from build123d import *

# Parameters (mm, degrees)
SKETCH018_W     = 50
SKETCH018_H     = 18
PAD011_DEPTH    = 4.5
SKETCH019_R     = 1.3375
POCKET006_DEPTH = 8
POCKET007_DEPTH = 9.001
SKETCH053_R     = 1.3375
SKETCH053_R_2   = 2.5
PAD029_DEPTH    = 6.5
SKETCH055_W     = 8.5
SKETCH055_H     = 1
SKETCH055_W_2   = 24
POCKET024_DEPTH = 1


with BuildPart() as part:
    # Sketch018 → Pad011 (new body, symmetric)
    with BuildSketch(Plane.XY):
        with Locations((25, 9)):
            Rectangle(SKETCH018_W, SKETCH018_H)
    extrude(amount=PAD011_DEPTH, both=True)

    # Sketch019 → Pocket006 (cut)
    with BuildSketch(Plane.XZ):
        with Locations((5, 0)):
            Circle(SKETCH019_R)
        with Locations((25, 0)):
            Circle(SKETCH019_R)
        with Locations((45, 0)):
            Circle(SKETCH019_R)
    extrude(amount=-POCKET006_DEPTH, mode=Mode.SUBTRACT)

    # Sketch020 (on Face4 of Pocket006) → Pocket007 (cut, through all)
    with BuildSketch(Plane(origin=(0, 0, -4.5), x_dir=(1, 0, 0), z_dir=(0, 0, -1))):
        Polygon((0, -8), (43.5, -18), (0, -18), align=None)
    extrude(amount=-POCKET007_DEPTH, mode=Mode.SUBTRACT)

    # Sketch053 → Pad029 (join)
    with BuildSketch(Plane.YZ.offset(50)):
        Polygon((18, -4.5), (-6.5, -4.5), (-6.5, 4.5), (-15.5, 4.5), (-15.5, -4.5), (0, -24.5), (18, -24.5), align=None)
        with Locations((14, -7)):
            Circle(SKETCH053_R, mode=Mode.SUBTRACT)
        with Locations((4, -7)):
            Circle(SKETCH053_R, mode=Mode.SUBTRACT)
        with Locations((4, -22)):
            Circle(SKETCH053_R, mode=Mode.SUBTRACT)
        with Locations((14, -22)):
            Circle(SKETCH053_R, mode=Mode.SUBTRACT)
        with Locations((-11, 0)):
            Circle(SKETCH053_R_2, mode=Mode.SUBTRACT)
    extrude(amount=-PAD029_DEPTH)

    # Sketch055 (on Face7 of Pad029) → Pocket024 (cut)
    with BuildSketch(Plane.YZ.offset(50)):
        with Locations((13.75, -14.5)):
            Rectangle(SKETCH055_W, SKETCH055_H)
        with Locations((-3.5, -14.5)):
            Rectangle(SKETCH055_W_2, SKETCH055_H)
    extrude(amount=-POCKET024_DEPTH, mode=Mode.SUBTRACT)


with BuildPart() as part_1:
    # Body005 placement: moved
    add(part.part.moved(Location((75, 6.5, 0))))


solid = part_1.part
Work out the finished part from the listing and answer in its coordinate system (mm). A direction names the side the tool comes from. Coordinates: 2 decimals unless noted, no trailing zeros. Write each loop counter-clockwise with the first axis right and the second up, starting at its lowest first coordinate (ties: lowest second). Pieces come first, ordered by that corner, then holes. Notation, with made-up numbers: M 20.25,7.5 L 25.25,7.5 A33 ccw 25.25,40.5 Z; hole C -25,59 d1. An arc over 180 degrees is marked long. Write item = value, one per line.
1. The part is cut by section D-D (x = 120). Determine the outline of the cut face in (y, z) (1 decimal), then the cut area to 3 significant figures.
Solution:
outline = M -9,-4.5 L 6.5,-24.5 L 24.5,-24.5 L 24.5,4.5 L 6.5,4.5 L 6.5,1.3 L 14.5,1.3 L 14.5,-1.3 L 6.5,-1.3 L 6.5,-4.5 L 0,-4.5 L 0,4.5 L -9,4.5 Z; hole C -4.5,0 d5; hole C 10.5,-22 d2.7; hole C 10.5,-7 d2.7; hole C 20.5,-22 d2.7; hole C 20.5,-7 d2.7
area = 694 mm2
2. For faces 4 (the face through (101, 14, -4.5)), 5 (the face through (81.276, 10.444, 0.402)), 6 (the face through (122, 3, -4.5)), 7 (the face through (120, 14.5, 0)), 8 (the face through (96.45, 19.43, -0.06)), determine the directions among +Z, -Z, +X, -X, +Y, -Y from which every point of the face is accessible in a straight line to the end or side of a thin tool.
Solution:
face_4 = -Z, -X, +Y, -Y
face_5 = -Y
face_6 = +Z, +X, -X
face_7 = none
face_8 = +Z, -Z, -X, +Y
3. The part is cut by section B-B (y = 13.5). Determine the outline of the cut face in (x, z) (1 decimal), then the cut area to 3 significant figures.
Solution:
outline = M 75,-4.5 L 118.5,-4.5 L 118.5,-24.5 L 125,-24.5 L 125,-15 L 124,-15 L 124,-14 L 125,-14 L 125,4.5 L 75,4.5 Z; hole C 80,0 d2.7; hole C 100,0 d2.7; hole C 120,0 d2.7
area = 562 mm2
4. Flat-ended cylindrical pins translate along their axes: pin 1 (3.5 mm diameter, centred on x = 80, z = 0, fed in from +Y); pin 2 (0.5 mm diameter, centred on x = 124.5, z = -14.5, fed in from +Y); pin 3 (2.5 mm diameter, centred on x = 95.5, z = -2, fed in from -Y). Find the tip coordinate at first contact, or state that the pin passes through.
Solution:
pin_1 = 16.05
pin_2 = 16
pin_3 = 6.5
5. The part is cut by section C-C (z = -7). Determine the outline of the cut face in (x, y).
Solution:
outline = M 118.5,-7.06 L 125,-7.06 L 125,9.16 L 118.5,9.16 Z; M 118.5,11.84 L 125,11.84 L 125,19.16 L 118.5,19.16 Z; M 118.5,21.84 L 125,21.84 L 125,24.5 L 118.5,24.5 Z
6. The part is cut by section A-A (y = 20.5). Determine the outline of the cut face in (x, z).
Solution:
outline = M 101.1,-4.5 L 118.5,-4.5 L 118.5,-5.66 L 125,-5.66 L 125,4.5 L 101.1,4.5 Z; M 118.5,-24.5 L 125,-24.5 L 125,-23.34 L 118.5,-23.34 Z; M 118.5,-20.66 L 125,-20.66 L 125,-15 L 124,-15 L 124,-14 L 125,-14 L 125,-8.34 L 118.5,-8.34 Z
7. Straight lines are drawn through the part: line 1 (Z direction, x = 121.5, y = 10.5); line 2 (Z direction, x = 120, y = 13.25); line 3 (Z direction, x = 80, y = 12). For each, find the intervals that lie inside material, in ascending order. Write a range as from..to.
Solution:
line_1 = -24.5..-23.34, -20.66..-8.34, -5.66..4.5
line_2 = -24.5..-1.34, 1.34..4.5
line_3 = -4.5..-1.34, 1.34..4.5
8. Determine the mould class of faces 1 (the face through (121.8, -1.36, -14.36)), 2 (the face through (118.664, 10.444, 0.059)), 3 (the face through (118.5, 8, -13)) for opening direction X: released by +X, released by -X, zero draft, split by the parting line, or undercut.
Solution:
face_1 = zero draft
face_2 = undercut
face_3 = released by -X
